```python
from build123d import *

# Parameters (mm, degrees)
F0_W     = 189.5
F0_H     = 63
F1_DEPTH = 2


with BuildPart() as f1:
    # F0 (on Top) → F1 (new body)
    with BuildSketch(Plane.XY):
        Polygon((96.5, 73), (-103, 73), (-103, 51), (-105, 51), (-105, 29), (-103, 29), (-103, 0), (96.5, 0), (96.5, 29), (98.5, 29), (98.5, 51), (96.5, 51), align=None)
        with Locations((-3.25, 36.5)):
            Rectangle(F0_W, F0_H, mode=Mode.SUBTRACT)
    extrude(amount=F1_DEPTH)


solid = f1.part
```
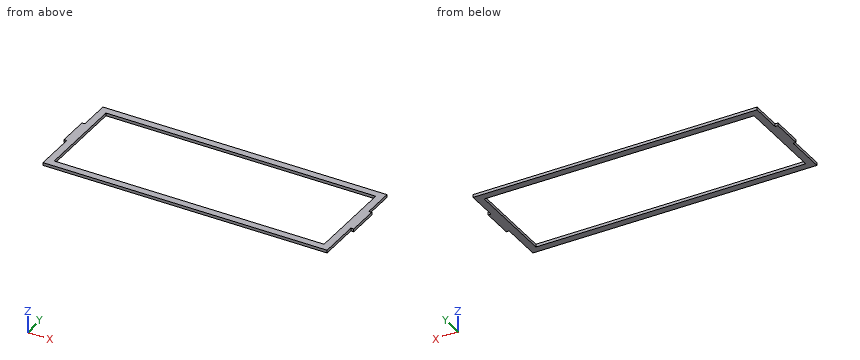
The listing builds one solid part. Answer for the finished solid, in the listing's coordinates (mm). Coordinates: 2 decimals unless noted, no trailing zeros. Loops run counter-clockwise (first coordinate to the right, second up) from the corner with the lowest first, then second, coordinate; pieces in that order, holes last. Notation, with made-up numbers: M 15.25,-35.75 L 70.25,-35.75 A16 ccw 70.25,-29.75 Z; hole C 53.25,-22.5 d8. An arc over 180 degrees is marked long. Answer as a JSON object with one key per item and string values. Group by question number.
Item 1: Section C-C (y = 56) is taken. Write down the section's boundary in (x, z), and give its area (3 significant figures).
Item 2: Section A-A (x = 50) is taken. Write down the section's boundary in (y, z), and give its area (3 significant figures).
Item 3: Section B-B (z = 1.25) is taken. Write down the section's boundary in (x, y).
Item 4: Each of these flat-tipped pins is pushed along its axis until it touches: P1, Ø1, axis at y = 64.5, z = 1, coming from the +X side; P2, Ø0.6, axis at x = 97.5, z = 1, coming from the +Y side; P3, Ø0.6, axis at x = 97.5, z = 0.5, coming from the -Y side. Where does it stop, or does it pass through?
Item 5: Consider L1, parallel to Y at x = -32.5, z = 1; L2, parallel to X at y = 17.5, z = 0.7; L3, parallel to X at y = 36, z = 1.45. Determine where each line is inside the solid, lowest interval first.
Solved:
{
 "1": {"outline": "M -103,0 L -98,0 L -98,2 L -103,2 Z; M 91.5,0 L 96.5,0 L 96.5,2 L 91.5,2 Z", "area": "20.0 mm2"},
 "2": {"outline": "M 0,0 L 5,0 L 5,2 L 0,2 Z; M 68,0 L 73,0 L 73,2 L 68,2 Z", "area": "20.0 mm2"},
 "3": {"outline": "M -105,29 L -103,29 L -103,0 L 96.5,0 L 96.5,29 L 98.5,29 L 98.5,51 L 96.5,51 L 96.5,73 L -103,73 L -103,51 L -105,51 Z; hole M -98,5 L 91.5,5 L 91.5,68 L -98,68 Z"},
 "4": {"P1": "stops at x = 96.5", "P2": "stops at y = 51", "P3": "stops at y = 29"},
 "5": {"L1": "y = 0 to 5, 68 to 73", "L2": "x = -103 to -98, 91.5 to 96.5", "L3": "x = -105 to -98, 91.5 to 98.5"}
}
